```python
from build123d import *

# Parameters (mm, degrees)
F0_R     = 45
F1_DEPTH = 14


with BuildPart() as f1:
    # F0 (on Top) → F1 (new body)
    with BuildSketch(Plane.XY):
        with BuildLine():
            ThreePointArc((-34.8038087036, 48.8742764624), (-27.493376273, -53.3302377747), (60, 0))
            ThreePointArc((60, 0), (53.4404878242, 27.2784578213), (35.1961912964, 48.5924697688))
            Line((35.1961912964, 48.5924697688), (-34.8038087036, 48.5924697688))
            Line((-34.8038087036, 48.5924697688), (-34.8038087036, 48.8742764624))
        make_face()
        Circle(F0_R, mode=Mode.SUBTRACT)
        with BuildLine():
            Line((-34.8038087036, 48.5924697688), (35.1961912964, 48.5924697688))
            ThreePointArc((35.1961912964, 48.5924697688), (0.2415466371, 59.9995137915), (-34.8038087036, 48.8742764624))
            Line((-34.8038087036, 48.8742764624), (-34.8038087036, 48.5924697688))
        make_face()
        with BuildLine():
            ThreePointArc((-34.8038087036, 48.8742764624), (0.2415466371, 59.9995137915), (35.1961912964, 48.5924697688))
            Line((35.1961912964, 48.5924697688), (35.1961912964, 66.2418827415))
            Line((35.1961912964, 66.2418827415), (21.3984008878, 66.2418827415))
            Line((21.3984008878, 66.2418827415), (-20.8038087036, 66.2418827415))
            Line((-20.8038087036, 66.2418827415), (-34.8038087036, 66.2418827415))
            Line((-34.8038087036, 66.2418827415), (-34.8038087036, 48.8742764624))
        make_face()
        Polygon((21.3984008878, 66.2418827415), (35.1961912964, 66.2418827415), (35.1961912964, 106.2418827415), (10.1961912964, 106.2418827415), (10.1961912964, 86.2418827415), (21.1961912964, 86.2418827415), align=None)
        Polygon((-34.8038087036, 106.2418827415), (-34.8038087036, 66.2418827415), (-20.8038087036, 66.2418827415), (-20.8038087036, 86.2418827415), (-9.8038087036, 86.2418827415), (-9.8038087036, 106.2418827415), align=None)
    extrude(amount=F1_DEPTH)


solid = f1.part
```
Work out the finished part from the listing and answer in its coordinate system (mm). A direction names the side the tool comes from. Round coordinates to 2 decimals unless told otherwise and drop trailing zeros. Loops run counter-clockwise (first coordinate to the right, second up) from the corner with the lowest first, then second, coordinate; pieces in that order, holes last. Notation, with made-up numbers: M 62.25,-37.75 L 98.25,-37.75 A10 cw 98.25,-28.75 Z; hole C 87.5,41.25 d5. An arc over 180 degrees is marked long. One line per question, with ' | ' between items.
Q1. Each of these flat-tipped pins is pushed along its axis until it touches: pin 1 Ø4 at (y, z) = (97.5, 8) entering from -X; pin 2 Ø8 at (x, z) = (19, 5) entering from -Y; pin 3 Ø4 at (x, z) = (4, 4.5) entering from +Y. Where does it stop, or does it pass through?
Conclusion:
pin 1: stops at x = -34.8 | pin 2: stops at y = -58.09 | pin 3: stops at y = 66.24
Q2. The mould has two halves that part along Y. Classify faces 1 (the flat face through (-20.804, 76, 7)), 2 (the flat face through (-22, 106.242, 7)), 3 (the flat face through (-34.804, 78, 7)): +Y half, -Y half, draft (parallel to the pull), parting line (faces both ways), or undercut.
Conclusion:
face 1: undercut | face 2: +Y half | face 3: draft
Q3. A tool of negligible diameter and unlimited length cuts with its end or side. For faces 4 (the flat face through (-14, 43, 14)), 5 (the flat face through (1, 66.242, 7)), 6 (the flat face through (10.196, 96, 7)), 7 (the flat face through (35.196, 77, 7)), 8 (the flat face through (-14, 43, 0)), from which of +Z, -Z, +X, -X, +Y, -Y can it reach the whole face along a straight path? Write none if from no direction.
Conclusion:
face 4: +Z, +X, -X, +Y, -Y | face 5: +Z, -Z | face 6: +Z, -Z, +Y | face 7: +Z, -Z, +X, +Y | face 8: -Z, +X, -X, +Y, -Y
Q4. Find section C-C, the plane y = 36. Give the vertices of the cut face in (x, z), then the cut area to 3 significant figures.
Conclusion:
outline: M -48,0 L -27,0 L -27,14 L -48,14 Z; M 27,0 L 48,0 L 48,14 L 27,14 Z | area: 588 mm2
Q5. Consider line 1 along X through (y, z) = (98.5, 11.25); line 2 along Y through (x, z) = (0, 7.25); line 3 along X through (y, z) = (85, 10.25). Determine where each line is inside the solid, lowest interval first. Write a range as from..to.
Conclusion:
line 1: x = -34.8..-9.8, 10.2..35.2 | line 2: y = -60..-45, 45..66.24 | line 3: x = -34.8..-20.8, 21.21..35.2
Q6. Find section D-D, the plane x = 48.5. Give the vertices of the cut face in (y, z), then the cut area to 3 significant figures.
Conclusion:
outline: M -35.32,0 L 35.32,0 L 35.32,14 L -35.32,14 Z | area: 989 mm2
Q7. Find section B-B, the plane z = 3. Give the vertices of the cut face in (x, y), then the cut area to 3 significant figures.
Conclusion:
outline: M -34.8,48.87 A60 ccw long 35.2,48.59 L 35.2,106.24 L 10.2,106.24 L 10.2,86.24 L 21.2,86.24 L 21.4,66.24 L -20.8,66.24 L -20.8,86.24 L -9.8,86.24 L -9.8,106.24 L -34.8,106.24 Z; hole C 0,0 d90 | area: 7,200 mm2
Q8. Find section A-A, the plane x = 0. Give the vertices of the cut face in (y, z), then the cut area to 3 significant figures.
Conclusion:
outline: M -60,0 L -45,0 L -45,14 L -60,14 Z; M 45,0 L 66.24,0 L 66.24,14 L 45,14 Z | area: 507 mm2
